Here's how the part is built. I have some questions about the finished solid (model axes, mm). Face numbers are marked on the shaded views. A direction names the side the tool comes from. Round coordinates to 2 decimals unless told otherwise and drop trailing zeros. Loops run counter-clockwise (first coordinate to the right, second up) from the corner with the lowest first, then second, coordinate; pieces in that order, holes last. Notation, with made-up numbers: M -17.5,12 L 41.5,12 A7 cw 41.5,20 Z; hole C -26.75,-35 d7. An arc over 180 degrees is marked long. Use a Markdown table: item, result.
```python
from build123d import *

# Parameters (mm, degrees)
SKETCH1_R           = 8.509
SKETCH1_R_2         = 5.334
BOSS_EXTRUDE1_DEPTH = 6.35
SKETCH2_R           = 7.747
SKETCH2_R_2         = 6.731
CUT_EXTRUDE1_DEPTH  = 2.54
BOSS_EXTRUDE2_DEPTH = 6.35


with BuildPart() as part:
    # Sketch1 → Boss-Extrude1 (new body)
    with BuildSketch(Plane.XY):
        Circle(SKETCH1_R)
        Circle(SKETCH1_R_2, mode=Mode.SUBTRACT)
    extrude(amount=BOSS_EXTRUDE1_DEPTH)

    # Sketch2 → Cut-Extrude1 (cut)
    with BuildSketch(Plane.XY.offset(6.35)):
        Circle(SKETCH2_R)
        Circle(SKETCH2_R_2, mode=Mode.SUBTRACT)
    cut_extrude1 = extrude(amount=-CUT_EXTRUDE1_DEPTH, mode=Mode.SUBTRACT)

    # Sketch3 → Boss-Extrude2 (add)
    with BuildSketch(Plane.XY):
        with BuildLine():
            Line((-3.175, 7.894457296), (-3.175, 8.509))
            Line((-3.175, 8.509), (-4.641469684, 11.049))
            Line((-4.641469684, 11.049), (4.641469684, 11.049))
            Line((4.641469684, 11.049), (3.175, 8.509))
            Line((3.175, 8.509), (3.175, 7.894457296))
            ThreePointArc((3.175, 7.894457296), (0, 8.509), (-3.175, 7.894457296))
        make_face()
    boss_extrude2 = extrude(amount=BOSS_EXTRUDE2_DEPTH)

    # Mirror1: Boss-Extrude2 across plane
    add(boss_extrude2.mirror(Plane.ZX))

    # Mirror2: Cut-Extrude1 across plane
    add(cut_extrude1.mirror(Plane(origin=(0, 0, 3.175), x_dir=(1, 0, 0), z_dir=(0, 0, -1))), mode=Mode.SUBTRACT)


solid = part.part
```
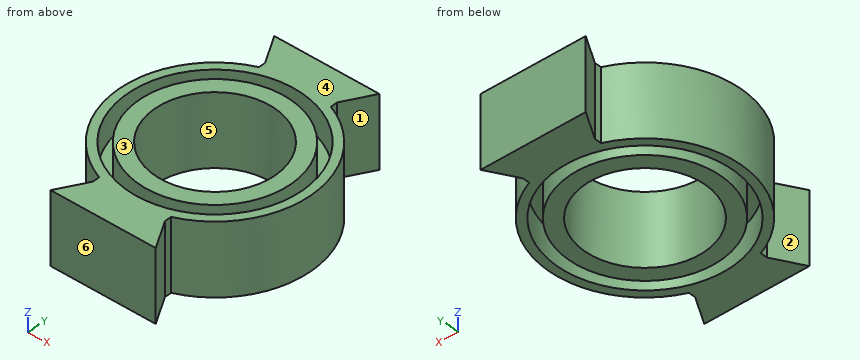
Q1. I need wall thicknesses on line 1 (Y direction, x = 0, z = 1.35); line 2 (X direction, y = 1.25, z = 6); line 3 (Y direction, x = 2.25, z = 1.25). Which ranges of each line are inside material? Lowest first, please. Write a range as from..to.
Return value:
| item | result |
|---|---|
| line 1 | y = -11.05..-7.75, -6.73..-5.33, 5.33..6.73, 7.75..11.05 |
| line 2 | x = -8.42..-7.65, -6.61..-5.19, 5.19..6.61, 7.65..8.42 |
| line 3 | y = -11.05..-7.41, -6.34..-4.84, 4.84..6.34, 7.41..11.05 |
Q2. Imagine slicing it at B-B, the plane z = 4.75. Please give me the cut outline in (x, y) (3 decimals).
Return value:
| item | result |
|---|---|
| outline | C 0,0 d13.462; M -4.641,-11.049 L 4.641,-11.049 L 3.175,-8.509 L 3.175,-7.894 A8.509 ccw 3.175,7.894 L 3.175,8.509 L 4.641,11.049 L -4.641,11.049 L -3.175,8.509 L -3.175,7.894 A8.509 ccw -3.175,-7.894 L -3.175,-8.509 Z; hole C 0,0 d15.494; hole C 0,0 d10.668 |
Q3. For the marked faces 1, 2 and 3, which set-ups out of +Z, -Z, +X, -X, +Y, -Y let a thin tool reach every point of the face, with its end or its side?
Return value:
| item | result |
|---|---|
| face 1 | +Z, -Z, +X |
| face 2 | +Z, -Z, -X |
| face 3 | +Z, +X, -X, +Y, -Y |
Q4. Imagine slicing it at A-A, the plane x = 0. Please give me the cut outline in (y, z), then the cut area to 3 significant figures.
Return value:
| item | result |
|---|---|
| outline | M -11.05,0 L -7.75,0 L -7.75,2.54 L -6.73,2.54 L -6.73,0 L -5.33,0 L -5.33,6.35 L -6.73,6.35 L -6.73,3.81 L -7.75,3.81 L -7.75,6.35 L -11.05,6.35 Z; M 5.33,0 L 6.73,0 L 6.73,2.54 L 7.75,2.54 L 7.75,0 L 11.05,0 L 11.05,6.35 L 7.75,6.35 L 7.75,3.81 L 6.73,3.81 L 6.73,6.35 L 5.33,6.35 Z |
| area | 62.3 mm^2 |
Q5. We'd pull the mould along Y, two halves only. Please class the marked faces 4, 5 and 6: pulls with the +Y half, pulls with the -Y half, needs draft (parallel to the pull), parting line crosses it, or undercut.
Return value:
| item | result |
|---|---|
| face 4 | needs draft |
| face 5 | undercut |
| face 6 | pulls with the -Y half |
Q6. Imagine slicing it at C-C, the plane y = 0. Please give me the cut outline in (x, z), then the cut area to 3 significant figures.
Return value:
| item | result |
|---|---|
| outline | M -8.51,0 L -7.75,0 L -7.75,2.54 L -6.73,2.54 L -6.73,0 L -5.33,0 L -5.33,6.35 L -6.73,6.35 L -6.73,3.81 L -7.75,3.81 L -7.75,6.35 L -8.51,6.35 Z; M 5.33,0 L 6.73,0 L 6.73,2.54 L 7.75,2.54 L 7.75,0 L 8.51,0 L 8.51,6.35 L 7.75,6.35 L 7.75,3.81 L 6.73,3.81 L 6.73,6.35 L 5.33,6.35 Z |
| area | 30.0 mm^2 |
Q7. Will these pins go through, and if not, where does the flat tip stop? P1, Ø1.5, axis at y = 1, z = 5.5, coming from the +X side; P2, Ø6, axis at x = 0.5, y = 2.5, coming from the +Z side; P3, Ø0.7, axis at y = -8.5, z = 4, coming from the -X side; P4, Ø0.5, axis at y = 8, z = 2, coming from the +X side.
Return value:
| item | result |
|---|---|
| P1 | stops at x = 8.51 |
| P2 | stops at z = 6.35 |
| P3 | stops at x = -3.37 |
| P4 | stops at x = 3.51 |
Q8. Imagine slicing it at D-D, the plane z = 3.25. Please give me the cut outline in (x, y) (3 decimals).
Return value:
| item | result |
|---|---|
| outline | M -4.641,-11.049 L 4.641,-11.049 L 3.175,-8.509 L 3.175,-7.894 A8.509 ccw 3.175,7.894 L 3.175,8.509 L 4.641,11.049 L -4.641,11.049 L -3.175,8.509 L -3.175,7.894 A8.509 ccw -3.175,-7.894 L -3.175,-8.509 Z; hole C 0,0 d10.668 |
